Geometry check sheet. Reference: drawing and pictorial views, mm from the part's lowest x, y, z. A direction names the side the tool comes from. Round coordinates to 2 decimals unless told otherwise and drop trailing zeros. Write each loop counter-clockwise with the first axis right and the second up, starting at its lowest first coordinate (ties: lowest second). Pieces come first, ordered by that corner, then holes. Notation, with made-up numbers: (29.5, 42.25) -> (77.5, 42.25) arc R27 cw to (77.5, 81.25) -> close; hole circle Ø9 at (-8.5, 75.5). An arc over 180 degrees is marked (long way). Write item = value, one per line.
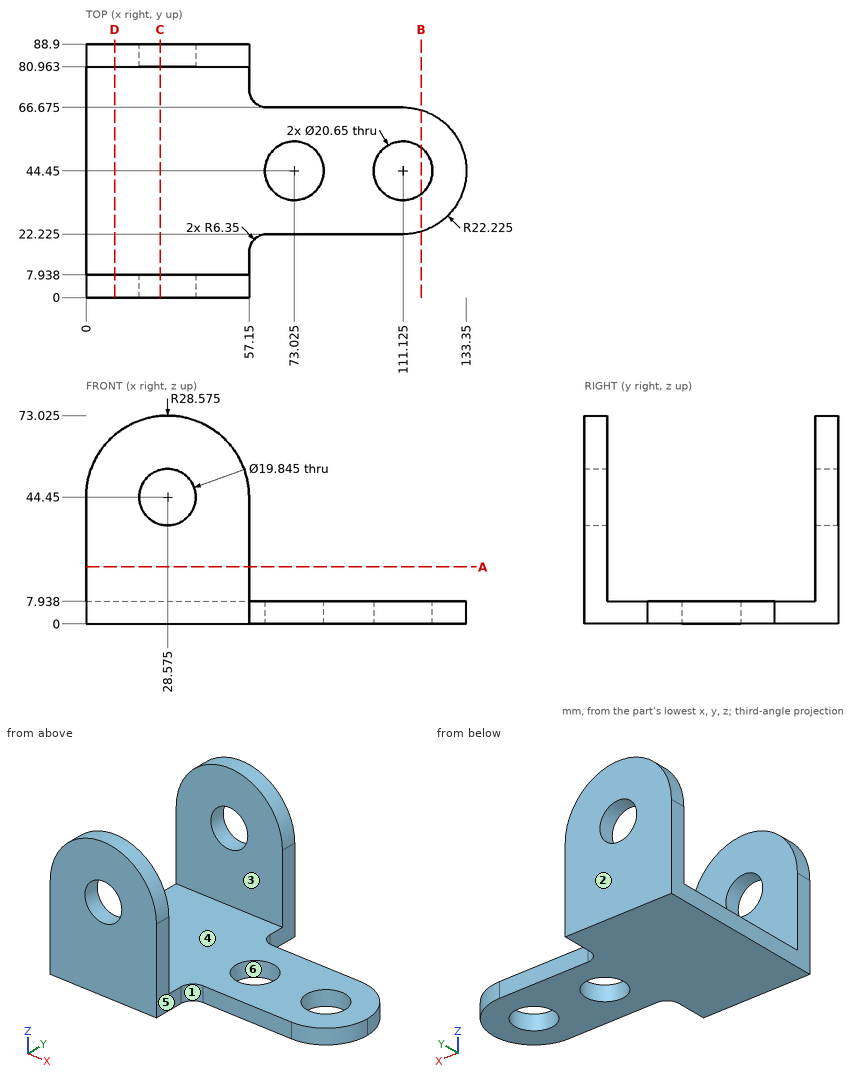
(1) Sectioned sample at D-D on x = 10. Enter the section's corners in (y, z) (1 decimal), then the cut area to 3 significant figures.
Worked answers:
outline = (0, 0) -> (88.9, 0) -> (88.9, 66.2) -> (81, 66.2) -> (81, 7.9) -> (7.9, 7.9) -> (7.9, 66.2) -> (0, 66.2) -> close
area = 1,630 mm²
(2) Go/stop test with flat-tipped pins: P1, Ø16, axis at x = 28.575, z = 44.45, coming from the +Y side; P2, Ø5, axis at y = 4.5, z = 23.5, coming from the +X side; P3, Ø4, axis at x = 85, z = 5, coming from the +Y side (1 decimal); P4, Ø8.5, axis at x = 98.5, z = 3, coming from the -Y side (1 decimal). Record where each tip stops, or that it passes through.
Worked answers:
P1 = through
P2 = 57.15
P3 = 66.7
P4 = 22.2
(3) Sectioned sample at B-B on x = 117.5. Enter the section's corners in (y, z).
Worked answers:
outline = (23.16, 0) -> (36.33, 0) -> (36.33, 7.94) -> (23.16, 7.94) -> close; (52.57, 0) -> (65.74, 0) -> (65.74, 7.94) -> (52.57, 7.94) -> close
(4) Material ranges on L1, parallel to X at y = 44.45, z = 5.5; L2, parallel to X at y = 3, z = 44.45; L3, parallel to X at y = 44, z = 4 (1 decimal), recorded low to high. Write a range as [from, to].
Worked answers:
L1 = [0, 62.7], [83.35, 100.8], [121.45, 133.35]
L2 = [0, 18.65], [38.5, 57.15]
L3 = [0, 62.7], [83.3, 100.8], [121.4, 133.3]
(5) Release check for a two-part mould opening along Y. For the marked faces 1, 2 and 3 record: pulls with the +Y half, pulls with the -Y half, needs draft (parallel to the pull), parting line crosses it, or undercut.
Worked answers:
face_1 = pulls with the -Y half
face_2 = pulls with the +Y half
face_3 = undercut
(6) Access from +Z, -Z, +X, -X, +Y, -Y to the whole of each face (thin tool, end or side, straight path). Record for the marked faces 4, 5 and 6.
Worked answers:
face_4 = +Z, +X, -X
face_5 = +Z, -Z, +X, -Y
face_6 = +Z, -Z
(7) Sectioned sample at C-C on x = 26. Enter the section's corners in (y, z), then the cut area to 3 significant figures.
Worked answers:
outline = (0, 0) -> (88.9, 0) -> (88.9, 34.87) -> (80.96, 34.87) -> (80.96, 7.94) -> (7.94, 7.94) -> (7.94, 34.87) -> (0, 34.87) -> close; (0, 54.03) -> (7.94, 54.03) -> (7.94, 72.91) -> (0, 72.91) -> close; (80.96, 54.03) -> (88.9, 54.03) -> (88.9, 72.91) -> (80.96, 72.91) -> close
area = 1,430 mm²
(8) Sectioned sample at A-A on z = 20. Enter the section's corners in (x, y).
Worked answers:
outline = (0, 0) -> (57.15, 0) -> (57.15, 7.94) -> (0, 7.94) -> close; (0, 80.96) -> (57.15, 80.96) -> (57.15, 88.9) -> (0, 88.9) -> close
